The figure shows three views and two pictorial views of one solid part (mm, origin at its lowest corner). Answer the questions. A direction names the side the tool comes from. Round coordinates to 2 decimals unless told otherwise and drop trailing zeros. Order: outer loops, then holes, each group sorted by start corner. A loop starts at its lowest first (then second) coordinate and runs counter-clockwise, first axis right, second up. Notation, with made-up numbers: (28, 33.5) - (74, 33.5) arc R9 ccw to (74, 42.5) - close; hole circle Ø2 at (12, 87.25). An arc over 180 degrees is marked (long way). Answer in a Markdown table with one row per item.
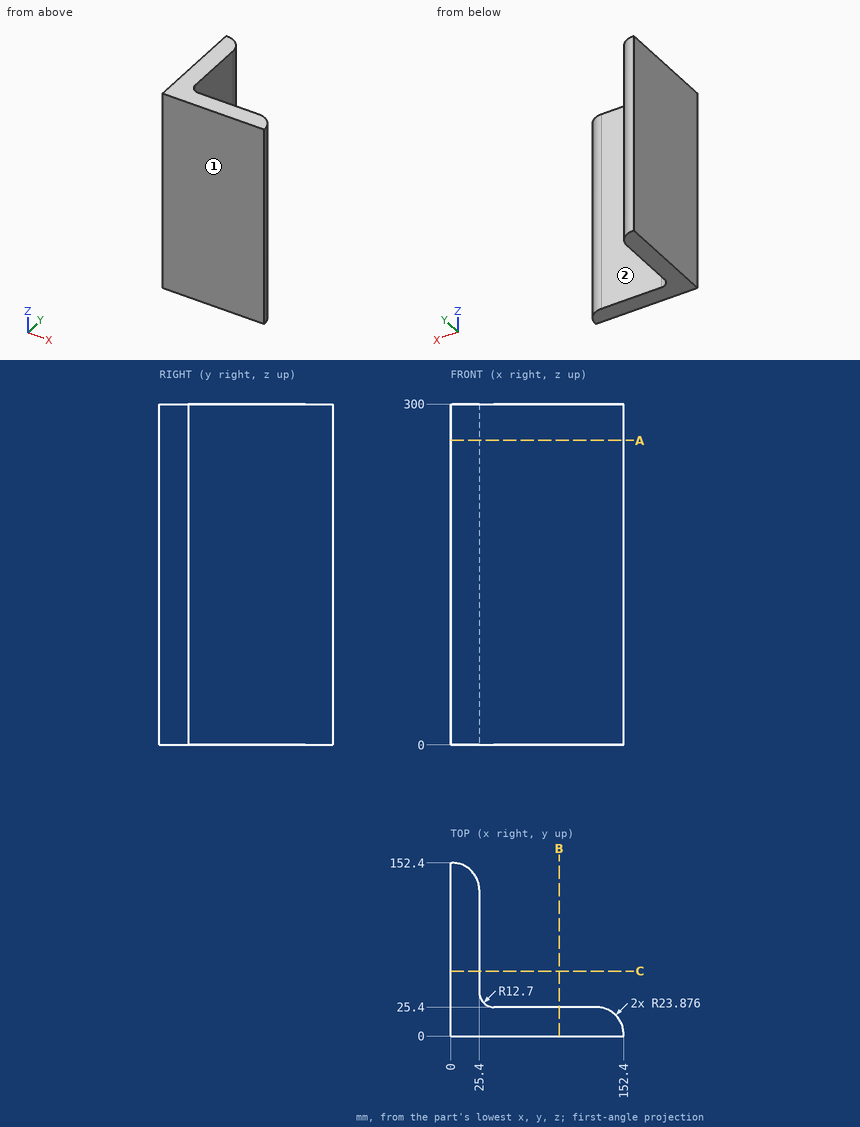
1) Find section B-B, the plane x = 95.5. Give the vertices of the cut face in (y, z), then the cut area to 3 significant figures.
Filled in:
| item | result |
|---|---|
| outline | (0, 0) - (25.4, 0) - (25.4, 300) - (0, 300) - close |
| area | 7,620 mm^2 |
2) Which of the six approach directions +Z, -Z, +X, -X, +Y, -Y give full straight-line access (tool end or side, diameter ignored) to the marked faces 1 and 2?
Filled in:
| item | result |
|---|---|
| face 1 | +Z, -Z, +X, -X, -Y |
| face 2 | +Z, -Z, +X, +Y |
3) Find section A-A, the plane z = 268. Give the vertices of the cut face in (x, y), then the cut area to 3 significant figures.
Filled in:
| item | result |
|---|---|
| outline | (0, 0) - (152.4, 0) - (152.4, 1.52) arc R23.88 ccw to (128.52, 25.4) - (38.1, 25.4) arc R12.7 cw to (25.4, 38.1) - (25.4, 128.52) arc R23.88 ccw to (1.52, 152.4) - (0, 152.4) - close |
| area | 6,890 mm^2 |
4) Each of these flat-tipped pins is pushed along its axis until it touches: pin 1 (1.5 mm diameter, centred on x = 79, z = 103, fed in from +Y); pin 2 (5 mm diameter, centred on y = 88.5, z = 217, fed in from -X). Where does it stop, or does it pass through?
Filled in:
| item | result |
|---|---|
| pin 1 | stops at y = 25.4 |
| pin 2 | stops at x = 0 |
5) Find the intervals of material crossed by probe 1 along Y at (x, z) = (82, 150); probe 2 along Y at (x, z) = (15.5, 88), in increasing order. Write a range as from..to.
Filled in:
| item | result |
|---|---|
| probe 1 | y = 0..25.4 |
| probe 2 | y = 0..147.88 |
